Source: CAD feature listing. Evaluate the final solid. Frame: model axes, mm. A direction names the side the tool comes from. Give positions to 0.01 mm unless a question says otherwise; leave off trailing zeros. Order: outer loops, then holes, each group sorted by start corner. A loop starts at its lowest first (then second) coordinate and runs counter-clockwise, first axis right, second up.
Autodesk Inventor part; units mm, degrees
ref_plane "Start Plane" through (0, 0, 0) normal (0, 0, 1) x (1, 0, 0)
ref_plane "End Plane" through (0, 0, 2000) normal (0, 0, 1) x (1, 0, 0)
ref_plane "YZ Plane" through (0, 0, 0) normal (1, 0, 0) x (0, 1, 0)
ref_plane "Start Plane" through (0, 0, 0) normal (0, 0, 1) x (1, 0, 0)
ref_plane "End Plane" through (0, 0, 2000) normal (0, 0, 1) x (1, 0, 0)
sketch "Sketch" plane through (0, 0, 0) normal (0, 0, 1) x (1, 0, 0)
  line L0 (-2.75, 0) -> (-2.75, -52.3795)
  line L1 (-9.6366, -60.3016) -> (-31.5567, -63.3823)
  line L2 (-35, -67.3434) -> (-35, -70)
  line L3 (-35, -70) -> (0, -70)
  line L4 (-18.875, -70) -> (-18.875, -61.6) construction
  line L5 (-25.7112, 0) -> (34.2816, 0) construction
  line L6 (0, 40) -> (0, -70) construction
  line L7 (0, -48) -> (0, 64) construction
  line L8 (2.75, 0) -> (2.75, -52.3795)
  line L9 (9.6366, -60.3016) -> (31.5567, -63.3823)
  line L10 (35, -67.3434) -> (35, -70)
  line L11 (35, -70) -> (0, -70)
  line L12 (-2.75, 0) -> (2.75, 0) construction
  line L13 (-2.75, 0) -> (-2.75, 52.3795)
  line L14 (-9.6366, 60.3016) -> (-31.5567, 63.3823)
  line L15 (-35, 67.3434) -> (-35, 70)
  line L16 (-35, 70) -> (0, 70)
  line L17 (2.75, 0) -> (2.75, 52.3795)
  line L18 (9.6366, 60.3016) -> (31.5567, 63.3823)
  line L19 (35, 67.3434) -> (35, 70)
  line L20 (35, 70) -> (0, 70)
  arc A0 (-35, 67.3434) -> (-31.5567, 63.3823) centre (-31, 67.3434) ccw
  arc A1 (31.5567, 63.3823) -> (35, 67.3434) centre (31, 67.3434) ccw
  arc A2 (35, -67.3434) -> (31.5567, -63.3823) centre (31, -67.3434) ccw
  arc A3 (-31.5567, -63.3823) -> (-35, -67.3434) centre (-31, -67.3434) ccw
  arc A4 (-2.75, 52.3795) -> (-9.6366, 60.3016) centre (-10.75, 52.3795) ccw
  arc A5 (9.6366, 60.3016) -> (2.75, 52.3795) centre (10.75, 52.3795) ccw
  arc A6 (2.75, -52.3795) -> (9.6366, -60.3016) centre (10.75, -52.3795) ccw
  arc A7 (-9.6366, -60.3016) -> (-2.75, -52.3795) centre (-10.75, -52.3795) ccw
  line L21 (0, 98) -> (0, -98) construction
  line L22 (-50.0367, 0) -> (50.0367, 0) construction
  point P0 (-2.75, -59.3338)
  point P1 (-35, -63.8662)
  point P2 (2.75, -59.3338)
  point P3 (35, -63.8662)
  point P4 (18.875, -70)
  point P5 (18.875, -61.6)
  point P6 (-2.75, 59.3338)
  point P7 (-35, 63.8662)
  point P8 (-18.875, 70)
  point P9 (-18.875, 61.6)
  point P10 (2.75, 59.3338)
  point P11 (35, 63.8662)
  point P12 (18.875, 61.6)
  point P13 (18.875, 70)
  dimension "d1" = 2.2662
  dimension "d2" = 8.4
  dimension "d3" = 16.125
  dimension "d4" = 2.75
  dimension "d5" = 35
  dimension "d10" = 70
  dimension "d14" = 4
  dimension "d15" = 8
extrude "Body" add sketch "Sketch" along normal up to surface (2000 mm away) from surface at 0
sketch "Sketch3" plane through (0, 0, 0) normal (0, 0, 1) x (1, 0, 0)
  line L0 (0, 0) -> (10, 0)
ref_plane "Work Plane3" through (0, 0, 0) normal (0, -1, 0) x (1, 0, 0)
sketch "Sketch4" plane through (0, 0, 0) normal (0, -1, 0) x (1, 0, 0)
  line L0 (-2, 0) -> (12, 0)
  line L1 (-2, 2000) -> (12, 2000)
  dimension "d19" = 2000
equation "\"d2\" = G_T1"
equation "\"d3\" = G_C"
equation "\"d4\" = 0.5 * G_T"
equation "\"d5\" = 0.5 * G_W"
equation "\"d10\" = 0.5 * G_H"
equation "\"d14\" = G_ER"
equation "\"d15\" = G_IR"
equation "\"d6\" = G_L"
equation "\"G_W\" = 70"
equation "\"G_H\" = 140"
equation "\"G_T\" = 5.5"
equation "\"G_T1\" = 8.4"
equation "\"G_C\" = 16.125"
equation "\"G_NG\" = 0.140541"
equation "\"G_L\" = d19"
equation "\"G_ER\" = 0.5 * G_IR"
equation "\"G_IR\" = 8"
equation "\"G_OFFSET_START\" = 0"
equation "\"G_OFFSET_END\" = 0"
properties part number "ISO 657/15 - SB 140x15 - 2000" material "Steel, Mild"
1) Reachability of faces 1 (the flat face through (2.75, 1, 986)), 2 (the flat face through (0, 0, 0)) from +Z, -Z, +X, -X, +Y, -Y: full face, straight path, thin tool, end or side. Return the list, or none.
Report:
face 1: +Z, -Z, +X
face 2: -Z, +X, -X, +Y, -Y
2) Draft query along Y for faces 3 (the flat face through (0, -70, 986)), 4 (the flat face through (0, 70, 986)), 5 (the flat face through (-2.75, 1, 986)), 6 (the flat face through (0, 0, 2000)). Return one class per face: +Y half, -Y half, draft (parallel to the pull), parting line (faces both ways), or undercut.
Report:
face 3: -Y half
face 4: +Y half
face 5: undercut
face 6: draft
3) Pin query (flat end, axial travel): pin 1 (6 mm diameter, centred on y = -0.5, z = 226, fed in from -X); pin 2 (2 mm diameter, centred on y = 4.5, z = 1111.5, fed in from +X). Return the tip coordinate at first contact, or that it passes through.
Report:
pin 1: stops at x = -2.75
pin 2: stops at x = 2.75
4) Material intervals for L1, parallel to Y at x = -30.5, z = 1861; L2, parallel to Y at x = -9, z = 407; L3, parallel to X at y = 46.5, z = 864, sorted ascending.
Report:
L1: y = -70 to -63.23, 63.23 to 70
L2: y = -70 to -60.19, 60.19 to 70
L3: x = -2.75 to 2.75
5) Section query A-A, the plane z = 235. Return the cut outline in (x, y), and give its area (3 significant figures).
Report:
outline: (-35, -70) - (35, -70) - (35, -67.34) arc R4 ccw to (31.56, -63.38) - (9.64, -60.3) arc R8 cw to (2.75, -52.38) - (2.75, 52.38) arc R8 cw to (9.64, 60.3) - (31.56, 63.38) arc R4 ccw to (35, 67.34) - (35, 70) - (-35, 70) - (-35, 67.34) arc R4 ccw to (-31.56, 63.38) - (-9.64, 60.3) arc R8 cw to (-2.75, 52.38) - (-2.75, -52.38) arc R8 cw to (-9.64, -60.3) - (-31.56, -63.38) arc R4 ccw to (-35, -67.34) - close
area: 1,880 mm2
6) Section query B-B, the plane y = 32. Return the cut outline in (x, z).
Report:
outline: (-2.75, 0) - (2.75, 0) - (2.75, 2000) - (-2.75, 2000) - close
